Design review of the part built by this model. Coordinates are the model's own, in mm. A direction names the side the tool comes from. Coordinates: 2 decimals unless noted, no trailing zeros. Loops run counter-clockwise (first coordinate to the right, second up) from the corner with the lowest first, then second, coordinate; pieces in that order, holes last.
from build123d import *

# Parameters (mm, degrees)
PAD_DEPTH                  = 1.28
SKETCH005_W                = 145
SKETCH005_H                = 1.6
SKETCH005_W_2              = 82.424179
PAD003_DEPTH               = 5
PAD004_DEPTH               = 1.28
PAD004_MIRRORED_2_DEPTH    = 1.28
LINEARPATTERN_COUNT        = 3
LINEARPATTERN_PITCH        = 51.5
PAD005_DEPTH               = 1.28
PAD005_MIRRORED001_2_DEPTH = 1.28
LINEARPATTERN001_COUNT     = 4
LINEARPATTERN001_PITCH     = 40.3390943124


with BuildPart() as part:
    # Sketch → Pad (new body)
    with BuildSketch(Plane.XZ):
        Polygon((0, 0), (0, 110), (-160, 110), (-90, 0), align=None)
    extrude(amount=-PAD_DEPTH)

    # Sketch005 (on Face6 of Pad) → Pad003 (join)
    with BuildSketch(Plane(origin=(0, 1.28, 0), x_dir=(1, 0, 0), z_dir=(0, 1, 0))):
        with Locations((-77.5, -105.0479535608)):
            Rectangle(SKETCH005_W, SKETCH005_H)
        with Locations((-46.2120895, -5.171919)):
            Rectangle(SKETCH005_W_2, SKETCH005_H)
    extrude(amount=PAD003_DEPTH)

    # Sketch006 (on Face5 of Pad003) → Pad004 (join)
    with BuildSketch(Plane(origin=(0, 1.28, 0), x_dir=(1, 0, 0), z_dir=(0, 1, 0))):
        with BuildLine():
            Line((0, -110), (0, -106.5))
            Line((0, -106.5), (1, -106.5))
            ThreePointArc((1, -106.5), (2.7, -108.2), (4.4, -106.5))
            Line((4.4, -106.5), (6.2, -106.5))
            ThreePointArc((2.6999832282, -110), (5.1748678044, -108.9748796639), (6.2, -106.5))
            Line((0, -110), (2.6999832282, -110))
        make_face()
    pad004 = extrude(amount=-PAD004_DEPTH)

    # Sketch006 Mirrored 2 → Pad004 Mirrored 2 (add)
    with BuildSketch(Plane(origin=(0, 1.28, 213), x_dir=(1, 0, 0), z_dir=(0, -1, 0))):
        with BuildLine():
            Line((0, -110), (0, -106.5))
            Line((0, -106.5), (1, -106.5))
            ThreePointArc((1, -106.5), (2.7, -108.2), (4.4, -106.5))
            Line((4.4, -106.5), (6.2, -106.5))
            ThreePointArc((2.6999832282, -110), (5.1748678044, -108.9748796639), (6.2, -106.5))
            Line((0, -110), (2.6999832282, -110))
        make_face()
    pad004_mirrored_2 = extrude(amount=PAD004_MIRRORED_2_DEPTH)

    # LinearPattern: Pad004, Pad004 Mirrored 2 ×3
    with Locations(*[(0, 0, -i * LINEARPATTERN_PITCH) for i in range(1, LINEARPATTERN_COUNT)]):
        add(pad004)
        add(pad004_mirrored_2)

    # Sketch007 (on Face5 of Pad003) → Pad005 (join)
    with BuildSketch(Plane(origin=(0, 1.28, 0), x_dir=(1, 0, 0), z_dir=(0, 1, 0))):
        with BuildLine():
            Line((-160, -110), (-158.1209357773, -107.0471847929))
            Line((-158.1209357773, -107.0471847929), (-158.9645972651, -106.5103093007))
            ThreePointArc((-161.8330463233, -104.6849326273), (-161.3115101309, -107.0318454932), (-158.9645972651, -106.5103093007))
            Line((-161.8330463233, -104.6849326273), (-163.3516370013, -103.7185567413))
            ThreePointArc((-163.3516370013, -103.7185567413), (-163.8154739704, -106.3568889713), (-162.2778663036, -108.5504487158))
            Line((-160, -110), (-162.2778663036, -108.5504487159))
        make_face()
    pad005 = extrude(amount=-PAD005_DEPTH)

    # Sketch007 Mirrored001 2 → Pad005 Mirrored001 2 (add)
    with BuildSketch(Plane(origin=(-188.1242244958, 1.28, 295.6237813506), x_dir=(0.4235294118, 0, 0.9058823529), z_dir=(0, -1, 0))):
        with BuildLine():
            Line((-160, -110), (-158.1209357773, -107.0471847929))
            Line((-158.1209357773, -107.0471847929), (-158.9645972651, -106.5103093007))
            ThreePointArc((-161.8330463233, -104.6849326273), (-161.3115101309, -107.0318454932), (-158.9645972651, -106.5103093007))
            Line((-161.8330463233, -104.6849326273), (-163.3516370013, -103.7185567413))
            ThreePointArc((-163.3516370013, -103.7185567413), (-163.8154739704, -106.3568889713), (-162.2778663036, -108.5504487158))
            Line((-160, -110), (-162.2778663036, -108.5504487159))
        make_face()
    pad005_mirrored001_2 = extrude(amount=PAD005_MIRRORED001_2_DEPTH)

    # LinearPattern001: Pad005, Pad005 Mirrored001 2 ×4
    with Locations(*[Vector(0.5368754922, 0, -0.8436614877) * (i * LINEARPATTERN001_PITCH) for i in range(1, LINEARPATTERN001_COUNT)]):
        add(pad005)
        add(pad005_mirrored001_2)


with BuildPart() as part_1:
    # Body placement: moved
    add(part.part.moved(Location((0, 55, 0))))


solid = part_1.part
Q1. Take a section at A-A, the plane y = 58.5. Write out the cut boundary in (x, z).
Q2. For line 1 (Z direction, x = 2.7, y = 55.3); line 2 (Z direction, x = -104, y = 58.5); line 3 (X direction, y = 55.9, z = 106.5), list the stretches that pass through material, from the lowest coordinate up.
Q3. Machinability: for faces 1 (the cylindrical face through (3.95, 55.65, 53.85)), 2 (the flat face through (-79, 59, 104.248)), which of the approach directions +Z, -Z, +X, -X, +Y, -Y give a long, thin tool a straight path to every point of the face, cutting with its end or side? Answer none if there is none.
Q4. Clearance check with flat-ended pins moving along their axes: pin 1 Ø1 at (x, y) = (2, 55.5) entering from -Z; pin 2 Ø0.8 at (y, z) = (59.5, 5) entering from -X; pin 3 Ø6 at (x, z) = (-91, 91) entering from +Y; pin 4 Ø3 at (y, z) = (57.5, 65.5) entering from +X. State where each tip first meets the part, or that it passes through.
Q5. Take a section at C-C, the plane z = 92.5. Write out the cut boundary in (x, y).
Q6. Take a section at B-B, the plane z = 81. Write out the cut boundary in (x, y), then the cut area to 3 significant figures.
Q7. The part is to be moulded in two halves that separate along Z. For faces 3 (the flat face through (-47, 59, 4.372)), 4 (the flat face through (-79, 59, 105.848)), 5 (the cylindrical face through (3.07, 55.65, 108.16)), say which applies: pulls with the +Z half, pulls with the -Z half, needs draft (parallel to the pull), parting line crosses it, or undercut.
Entries:
1. outline: (-150, 104.25) - (-5, 104.25) - (-5, 105.85) - (-150, 105.85) - close; (-87.42, 4.37) - (-5, 4.37) - (-5, 5.97) - (-87.42, 5.97) - close
2. line 1: z = 0 to 1.8, 5.2 to 7, 51.5 to 53.3, 56.7 to 58.5, 103 to 104.8, 108.2 to 110
2. line 2: z = 104.25 to 105.85
2. line 3: x = -163.78 to -161.84, -158.96 to 1, 4.4 to 6.2
3. face 1: +Y, -Y
3. face 2: +X, -X, +Y
4. pin 1: stops at z = 0
4. pin 2: stops at x = -87.42
4. pin 3: stops at y = 56.28
4. pin 4: stops at x = 0
5. outline: (-148.86, 55) - (0, 55) - (0, 56.28) - (-148.86, 56.28) - close
6. outline: (-141.55, 55) - (0, 55) - (0, 56.28) - (-141.55, 56.28) - close
6. area: 181 mm2
7. face 3: pulls with the -Z half
7. face 4: pulls with the +Z half
7. face 5: undercut
